from build123d import *

# Parameters (mm, degrees)
SKETCH1_R           = 16
BOSS_EXTRUDE1_DEPTH = 10
SKETCH2_R           = 18
SKETCH2_R_2         = 16
BOSS_EXTRUDE2_DEPTH = 12
SKETCH3_R           = 2
CUT_EXTRUDE1_DEPTH  = 10
CUT_EXTRUDE2_REACH  = 14
SKETCH4_R           = 3
CUT_EXTRUDE3_REACH  = 12
SKETCH5_R           = 2
FILLET1_R           = 5
BOSS_EXTRUDE3_START = -2
SKETCH7_R           = 16
SKETCH7_R_2         = 14
BOSS_EXTRUDE3_DEPTH = 2


with BuildPart() as part:
    # Sketch1 → Boss-Extrude1 (new body)
    with BuildSketch(Plane.XY):
        Polygon((-40, 83), (-70, 83), (-40, -7), (-40, -83), (40, -83), (40, -7), (10, 83), align=None)
        with Locations((-30, 60)):
            Circle(SKETCH1_R, mode=Mode.SUBTRACT)
    extrude(amount=BOSS_EXTRUDE1_DEPTH)

    # Sketch2 → Boss-Extrude2 (add)
    with BuildSketch(Plane.XY.offset(10)):
        with Locations((-30, 60)):
            Circle(SKETCH2_R)
        with Locations((-30, 60)):
            Circle(SKETCH2_R_2, mode=Mode.SUBTRACT)
    extrude(amount=-BOSS_EXTRUDE2_DEPTH)

    # Sketch3 → Cut-Extrude1 (cut)
    with BuildSketch(Plane.XY.offset(10)):
        with Locations((-25, -47)):
            Circle(SKETCH3_R)
        with Locations((15, -47)):
            Circle(SKETCH3_R)
    extrude(amount=-CUT_EXTRUDE1_DEPTH, mode=Mode.SUBTRACT)

    # Sketch4 → Cut-Extrude2 (cut, up to next)
    with BuildSketch(Plane.XY.offset(10), mode=Mode.PRIVATE) as cut_extrude2_sk1:
        with Locations((-57, 76)):
            Circle(SKETCH4_R)
    cut_extrude2_tool1 = extrude(cut_extrude2_sk1.sketch, amount=-CUT_EXTRUDE2_REACH, mode=Mode.PRIVATE) & part.part
    add(cut_extrude2_tool1.solids().sort_by_distance((-57, 76, 10))[0], mode=Mode.SUBTRACT)

    # Sketch5 → Cut-Extrude3 (cut, up to next)
    with BuildSketch(Plane(origin=(0, 0, 0), x_dir=(-1, 0, 0), z_dir=(0, 0, -1)), mode=Mode.PRIVATE) as cut_extrude3_sk1:
        with Locations((5, -50)):
            Circle(SKETCH5_R)
    cut_extrude3_tool1 = extrude(cut_extrude3_sk1.sketch, amount=-CUT_EXTRUDE3_REACH, mode=Mode.PRIVATE) & part.part
    add(cut_extrude3_tool1.solids().sort_by_distance((-5, -50, 0))[0], mode=Mode.SUBTRACT)

    # Fillet1
    fillet1_edges = [part.edges().sort_by_distance(p)[0] for p in [
        (-70, 83, 5),
        (10, 83, 5),
    ]]
    fillet(fillet1_edges, radius=FILLET1_R)

    # Sketch7 → Boss-Extrude3 (add)
    with BuildSketch(Plane.XY.offset(10).offset(BOSS_EXTRUDE3_START)):
        with Locations((-30, 60)):
            Circle(SKETCH7_R)
        with Locations((-30, 60)):
            Circle(SKETCH7_R_2, mode=Mode.SUBTRACT)
    extrude(amount=BOSS_EXTRUDE3_DEPTH)


solid = part.part
Input: part model. Units: mm. Frame: model coordinates. A direction names the side the tool comes from. Round coordinates to 2 decimals unless told otherwise and drop trailing zeros. Loops run counter-clockwise (first coordinate to the right, second up) from the corner with the lowest first, then second, coordinate; pieces in that order, holes last. Notation, with made-up numbers: (47.5, -30) -> (96.5, -30) arc R18 ccw to (96.5, -8) -> close; hole circle Ø11 at (24.5, 39). An arc over 180 degrees is marked (long way). Answer as a JSON object with one key per item and string values. Group by question number.
1) Reachability of faces 4 (the flat face through (-30.07, 45.85, 8)), 5 (the flat face through (-40, -44, 5)), 6 (the cylindrical face through (-67.157, 80.87, 5.07)) from +Z, -Z, +X, -X, +Y, -Y: full face, straight path, thin tool, end or side. Return the list, or none.
2) Section query D-D on y = 3.5. Output: boundary loops of the cut face in (x, z).
3) Pin query (flat end, axial travel): pin 1 (6 mm diameter, centred on x = -48.5, y = 14.5, fed in from -Z); pin 2 (2 mm diameter, centred on y = -3, z = 2, fed in from -X); pin 3 (5 mm diameter, centred on x = -57, y = 76, fed in from -Z); pin 4 (5 mm diameter, centred on y = -29, z = 6.5, fed in from -X). Return the tip coordinate at first contact, or that it passes through.
4) Draft query along X for faces 1 (the cylindrical face through (15, -49, 5)), 2 (the flat face through (40, -46, 5)), 3 (the flat face through (-54, 35, 5)). Return one class per face: +X half, -X half, draft (parallel to the pull), parting line (faces both ways), or undercut.
5) Section query A-A on x = -57. Output: boundary loops of the cut face in (y, z).
6) Ray query, L1, parallel to Y at x = -29, z = 6.75; L2, parallel to Z at x = 32, y = -52.5; L3, parallel to Y at x = -25, z = 3.25. Return the intervals inside material, ascending.
7) Section query C-C on x = -30. Output: boundary loops of the cut face in (y, z).
8) Section query B-B on z = 3.75. Output: boundary loops of the cut face in (x, y).
Reply:
{
 "1": {"face 4": "-Z", "face 5": "+Z, -Z, -X, -Y", "face 6": "+Z, -Z, -X"},
 "2": {"outline": "(-43.5, 0) -> (36.5, 0) -> (36.5, 10) -> (-43.5, 10) -> close"},
 "3": {"pin 1": "stops at z = 0", "pin 2": "stops at x = -41.67", "pin 3": "passes through", "pin 4": "stops at x = -40"},
 "4": {"face 1": "undercut", "face 2": "+X half", "face 3": "-X half"},
 "5": {"outline": "(44, 0) -> (73, 0) -> (73, 10) -> (44, 10) -> close; (79, 0) -> (83, 0) -> (83, 10) -> (79, 10) -> close"},
 "6": {"L1": "y = -83 to 44.03, 75.97 to 83", "L2": "z = 0 to 10", "L3": "y = -83 to -49, -45 to 44.8, 75.2 to 83"},
 "7": {"outline": "(-83, 0) -> (42, 0) -> (42, -2) -> (44, -2) -> (44, 8) -> (46, 8) -> (46, 10) -> (-83, 10) -> close; (74, 8) -> (76, 8) -> (76, -2) -> (78, -2) -> (78, 0) -> (83, 0) -> (83, 10) -> (74, 10) -> close"},
 "8": {"outline": "(-67.81, 76.42) -> (-40, -7) -> (-40, -83) -> (40, -83) -> (40, -7) -> (11.14, 79.58) arc R5 ccw to (6.4, 83) -> (-63.06, 83) arc R5 ccw to start; hole circle Ø6 at (-57, 76); hole circle Ø32 at (-30, 60); hole circle Ø4 at (-25, -47); hole circle Ø4 at (-5, -50); hole circle Ø4 at (15, -47)"}
}
